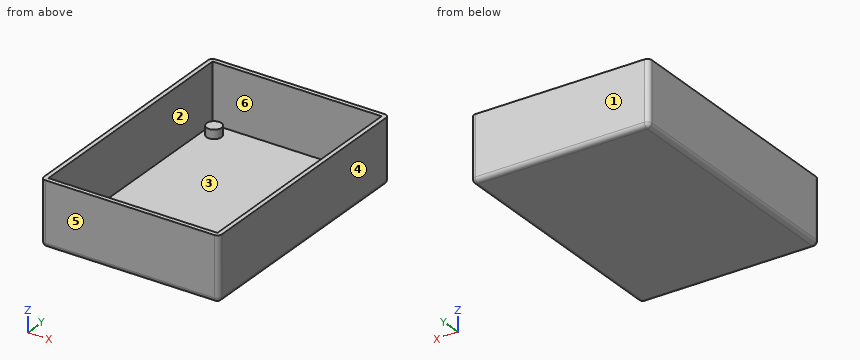
```python
from build123d import *

# Parameters (mm, degrees)
BOX_W        = 57
BOX_H        = 82
BOX_DEPTH    = 20
THICKNESS_T  = 1.5
SKETCH003_R  = 2.5
PAD001_DEPTH = 3


with BuildPart() as part:
    # Box → Box (new body)
    with BuildSketch(Plane.XY):
        with Locations((28.5, 41)):
            Rectangle(BOX_W, BOX_H)
    extrude(amount=BOX_DEPTH)

    # Thickness
    thickness_openings = [part.faces().sort_by_distance(p)[0] for p in [
        (28.5, 41, 20),
    ]]
    offset(amount=THICKNESS_T, openings=thickness_openings)


with BuildPart() as part_1:
    # Thickness placement: moved
    add(part.part.moved(Location((-1.5, 0, 0))))

    # Sketch003 → Pad001 (new body)
    with BuildSketch(Plane(origin=(-1.5, 0, 0), x_dir=(1, 0, 0), z_dir=(0, 0, 1))):
        with Locations((3.53528, 2.636141)):
            Circle(SKETCH003_R)
        with Locations((41.372181, 2.740742)):
            Circle(SKETCH003_R)
        with Locations((3.781813, 77.146011)):
            Circle(SKETCH003_R)
        with Locations((51.846909, 76.723869)):
            Circle(SKETCH003_R)
    extrude(amount=PAD001_DEPTH)


solid = part_1.part
```
Check sheet for the modelled part. Datum: model origin and axes. Units: mm. Face numbers are marked on the shaded views. A direction names the side the tool comes from. Give positions to 0.01 mm unless a question says otherwise; leave off trailing zeros. Write each loop counter-clockwise with the first axis right and the second up, starting at its lowest first coordinate (ties: lowest second). Pieces come first, ordered by that corner, then holes.
Item 1: Cross-section at B-B (x = 23). Enter the section's corners in (y, z), and give its area (3 significant figures).
Item 2: Cross-section at A-A (z = 13.5). Enter the section's corners in (x, y).
Item 3: Scan lines: L1, parallel to Y at x = 23.5, z = 2.75; L2, parallel to X at y = 25.5, z = 15.5; L3, parallel to Z at x = 7, y = 13. Record each from-to range of solid material in increasing order.
Item 4: Cross-section at C-C (y = 24). Enter the section's corners in (x, z).
Item 5: Cross-section at D-D (x = 49). Enter the section's corners in (y, z).
Item 6: Draft check along X on the marked faces 1, 2, 3 and 4. Enter one of: released by +X, released by -X, zero draft, split by the parting line, or undercut.
Item 7: Gauge pin test, flat ends, axial feed: pin 1 (8 mm diameter, centred on x = 23.5, y = 30.5, fed in from +Z); pin 2 (5.5 mm diameter, centred on x = 41, y = 3.5, fed in from +Z). Record the tip position at first contact, or that the pin passes through.
Item 8: Access from +Z, -Z, +X, -X, +Y, -Y to the whole of each face (thin tool, end or side, straight path). Record for the marked faces 5 and 6.
Report:
1. outline: (-1.5, 0) arc R1.5 ccw to (0, -1.5) - (82, -1.5) arc R1.5 ccw to (83.5, 0) - (83.5, 20) - (82, 20) - (82, 0) - (0, 0) - (0, 20) - (-1.5, 20) - close
1. area: 187 mm2
2. outline: (-3, 0) arc R1.5 ccw to (-1.5, -1.5) - (55.5, -1.5) arc R1.5 ccw to (57, 0) - (57, 82) arc R1.5 ccw to (55.5, 83.5) - (-1.5, 83.5) arc R1.5 ccw to (-3, 82) - close; hole (-1.5, 0) - (55.5, 0) - (55.5, 82) - (-1.5, 82) - close
3. L1: y = -1.5 to 0, 82 to 83.5
3. L2: x = -3 to -1.5, 55.5 to 57
3. L3: z = -1.5 to 0
4. outline: (-3, 0) arc R1.5 ccw to (-1.5, -1.5) - (55.5, -1.5) arc R1.5 ccw to (57, 0) - (57, 20) - (55.5, 20) - (55.5, 0) - (-1.5, 0) - (-1.5, 20) - (-3, 20) - close
5. outline: (-1.5, 0) arc R1.5 ccw to (0, -1.5) - (82, -1.5) arc R1.5 ccw to (83.5, 0) - (83.5, 20) - (82, 20) - (82, 0) - (78.83, 0) - (78.83, 3) - (74.62, 3) - (74.62, 0) - (0, 0) - (0, 20) - (-1.5, 20) - close
6. face 1: zero draft
6. face 2: undercut
6. face 3: undercut
6. face 4: released by +X
7. pin 1: stops at z = 0
7. pin 2: stops at z = 3
8. face 5: +Z, -Z, +X, -X, -Y
8. face 6: +Z
